The listing builds one solid part. Answer for the finished solid, in the listing's coordinates (mm). Coordinates: 2 decimals unless noted, no trailing zeros. Order: outer loops, then holes, each group sorted by start corner. A loop starts at its lowest first (then second) coordinate and runs counter-clockwise, first axis right, second up. Notation, with made-up numbers: (30, -33) -> (45, -33) arc R10 ccw to (45, -19) -> close; hole circle Ø3 at (56.25, -26.75). An arc over 180 degrees is marked (long way). Write item = value, one per line. Start each with the question number.
Autodesk Inventor part; units mm, degrees
ref_plane "YZ Plane" through (0, 0, 0) normal (1, 0, 0) x (0, 1, 0)
ref_plane "XZ Plane" through (0, 0, 0) normal (0, 1, 0) x (-1, 0, 0)
ref_plane "XY Plane" through (0, 0, 0) normal (0, 0, 1) x (1, 0, 0)
sketch "スケッチ1" plane through (0, 0, 0) normal (0, 0, 1) x (1, 0, 0)
  circle A0 centre (0, 0) radius 4
  dimension "d0" = 8
extrude "押し出し1" add sketch "スケッチ1" along normal blind 100
sketch "スケッチ2" plane through (0, 0, 100) normal (0, 0, 1) x (1, 0, 0)
  circle A0 centre (0, 0) radius 4
sketch "スケッチ3" plane through (0, 0, 0) normal (0, 0, -1) x (-1, 0, 0)
  circle A0 centre (0, 0) radius 4
extrude "押し出し3" add sketch "スケッチ3" along normal blind 40
extrude "押し出し4" add sketch "スケッチ2" along normal blind 30
properties part number "8mm軸_1"
Item 1: Section A-A, the plane z = -21.5 is taken. Give the vertices of the cut face in (x, y).
Item 2: Each of these flat-tipped pins is pushed along its axis until it touches: pin 1 (2 mm diameter, centred on x = 1.5, z = 49, fed in from -Y); pin 2 (1 mm diameter, centred on y = -1, z = 28.5, fed in from +X). Where does it stop, or does it pass through?
Item 3: Section B-B, the plane y = 2.5 is taken. Give the vertices of the cut face in (x, z), then the cut area to 3 significant figures.
Item 4: Section C-C, the plane x = 1.75 is taken. Give the vertices of the cut face in (y, z).
Item 5: Consider probe 1 along X at (y, z) = (-0.25, 23.5); probe 2 along Y at (x, z) = (0.5, 58); probe 3 along X at (y, z) = (-2, -16). Determine where each line is inside the solid, lowest interval first.
A:
q1.outline = circle Ø8 at (0, 0)
q2.pin_1 = -3.97
q2.pin_2 = 3.97
q3.outline = (-3.12, -40) -> (3.12, -40) -> (3.12, 130) -> (-3.12, 130) -> close
q3.area = 1,060 mm^2
q4.outline = (-3.6, -40) -> (3.6, -40) -> (3.6, 130) -> (-3.6, 130) -> close
q5.probe_1 = -3.99 to 3.99
q5.probe_2 = -3.97 to 3.97
q5.probe_3 = -3.46 to 3.46
